Can you work these out from the model? Positions are in its coordinate system, mm. Face numbers are marked on the shaded views. A direction names the side the tool comes from. Give positions to 0.01 mm unless a question says otherwise; leave off trailing zeros. Write each loop counter-clockwise with the first axis right and the second up, starting at its lowest first coordinate (ties: lowest second). Pieces come first, ordered by that corner, then holes. Notation, with made-up numbers: M 85,19.25 L 110,19.25 A17 ccw 110,36.25 Z; hole C 63,7.5 d1. An arc over 180 degrees is marked long. Write each question's results on one line, items separated by ' | '.
from build123d import *

# Parameters (mm, degrees)
F0_R     = 2.75
F1_DEPTH = 10
F3_DEPTH = 10
F4_F1_R  = 5
F4_F2_R  = 5
F4_F3_R  = 5
F4_F4_R  = 5


with BuildPart() as f1:
    # F0 (on Top) → F1 (new body)
    with BuildSketch(Plane.XY):
        with BuildLine():
            ThreePointArc((-4.25, 0), (0, 4.25), (4.25, 0))
            Line((4.25, 0), (4.25, 3.201806685))
            Line((4.25, 3.201806685), (2.2350018844, 6.8861790933))
            Line((2.2350018844, 6.8861790933), (2.2350018844, 10.8956433833))
            Line((2.2350018844, 10.8956433833), (2.2350018844, 20))
            Line((2.2350018844, 20), (-2.2350018844, 20))
            Line((-2.2350018844, 20), (-2.2350018844, 10.8956433833))
            Line((-2.2350018844, 10.8956433833), (-2.2350018844, 6.8861790933))
            Line((-2.2350018844, 6.8861790933), (-4.25, 3.201806685))
            Line((-4.25, 3.201806685), (-4.25, 0))
        make_face()
        with BuildLine():
            ThreePointArc((-4.25, 0), (0, -4.25), (4.25, 0))
            ThreePointArc((4.25, 0), (0, 4.25), (-4.25, 0))
        make_face()
        Circle(F0_R, mode=Mode.SUBTRACT)
    extrude(amount=F1_DEPTH)

    # F2 (on face) → F3 (cut)
    with BuildSketch(Plane(origin=(-2.2350018844, 0, 0), x_dir=(0, -1, 0), z_dir=(-1, 0, 0))):
        Polygon((-10.8234519139, 3.9840904064), (-6.8861790933, 10), (-20, 10), (-20, 5.9617315419), (-17.2440130264, 5.9617315419), (-17.2440130264, 3.9840904064), align=None)
    extrude(amount=-F3_DEPTH, mode=Mode.SUBTRACT)

    # F4: fillet of radius 5 on 6 edges, made by hand

    # F4_f1
    f4_f1_edges = [f1.edges().sort_by_distance(p)[0] for p in [
        (-4.25, 3.201806685, 5),
    ]]
    fillet(f4_f1_edges, radius=F4_F1_R)

    # F4_f2
    f4_f2_edges = [f1.edges().sort_by_distance(p)[0] for p in [
        (-2.2350018844, 6.8861790933, 5),
    ]]
    fillet(f4_f2_edges, radius=F4_F2_R)

    # F4_f3
    f4_f3_edges = [f1.edges().sort_by_distance(p)[0] for p in [
        (4.25, 3.201806685, 5),
    ]]
    fillet(f4_f3_edges, radius=F4_F3_R)

    # F4_f4
    f4_f4_edges = [f1.edges().sort_by_distance(p)[0] for p in [
        (2.2350018844, 6.8861790933, 5),
    ]]
    fillet(f4_f4_edges, radius=F4_F4_R)


solid = f1.part
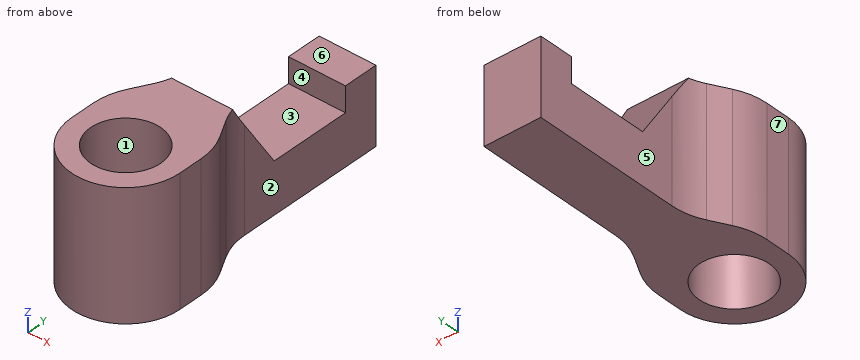
Item 1: I want a section at A-A, the plane x = 0. Please give me the cut outline in (y, z).
Geometry says:
outline: M -4.25,0 L -2.75,0 L -2.75,10 L -4.25,10 Z; M 2.75,0 L 20,0 L 20,5.96 L 17.24,5.96 L 17.24,3.98 L 10.82,3.98 L 6.89,10 L 2.75,10 Z
Item 2: I want a section at C-C, the plane z = 8.5. Please give me the cut outline in (x, y) (3 decimals), and give its area (3 significant figures).
Geometry says:
outline: M -4.25,0 A4.25 ccw 4.25,0 L 4.25,1.924 A5 ccw 3.637,4.323 L 2.848,5.765 A5 cw 2.244,7.868 L -2.244,7.868 A5 cw -2.848,5.765 L -3.637,4.323 A5 ccw -4.25,1.924 Z; hole C 0,0 d5.5 | area: 60.1 mm2
Item 3: Thinking about a two-plate mould opening in X: for the marked faces 1, 2 and 3, which applies, +X half, -X half, draft (parallel to the pull), parting line (faces both ways), or undercut?
Geometry says:
face 1: undercut | face 2: +X half | face 3: draft
Item 4: I want a section at D-D, the plane x = -1.75. Please give me the cut outline in (y, z), and give its area (3 significant figures).
Geometry says:
outline: M -3.87,0 L -2.12,0 L -2.12,10 L -3.87,10 Z; M 2.12,0 L 20,0 L 20,5.96 L 17.24,5.96 L 17.24,3.98 L 10.82,3.98 L 6.89,10 L 2.12,10 Z | area: 135 mm2
Item 5: For the marked faces 4, 5, 6 and 7, which set-ups out of +Z, -Z, +X, -X, +Y, -Y let a thin tool reach every point of the face, with its end or its side?
Geometry says:
face 4: +Z, +X, -X | face 5: +Z, -Z, -X, +Y | face 6: +Z, +X, -X, +Y | face 7: +Z, -Z, -X, +Y, -Y
Item 6: I'm going to push flat-ended pins straight in: pin 1 (2 mm diameter, centred on x = -0.5, y = 13, fed in from +Z); pin 2 (2.5 mm diameter, centred on y = 14.5, z = 2.5, fed in from +X) (3 decimals); pin 3 (2 mm diameter, centred on x = 2.5, z = 1, fed in from -Y). Where does each tip first touch, or does it pass through?
Geometry says:
pin 1: stops at z = 3.98 | pin 2: stops at x = 2.235 | pin 3: stops at y = -3.98
Item 7: I want a section at B-B, the plane y = -1.25. Please give me the cut outline in (x, z).
Geometry says:
outline: M -4.06,0 L -2.45,0 L -2.45,10 L -4.06,10 Z; M 2.45,0 L 4.06,0 L 4.06,10 L 2.45,10 Z
Item 8: If I drill on line 1 (X direction, y = 10, z = 4.75) (3 decimals); line 2 (Z direction, x = -2, y = 11); line 3 (Y direction, x = 1, z = 5.75), over which ranges is the centre line in solid material (lowest first)? Write a range as from..to.
Geometry says:
line 1: x = -2.235..2.235 | line 2: z = 0..3.98 | line 3: y = -4.13..-2.56, 2.56..9.67, 17.24..20
